```python
from build123d import *

# Parameters (mm, degrees)
BOSS_EXTRUDE1_DEPTH      = 4
BOSS_EXTRUDE1_DEPTH_BACK = 4
SKETCH3_W                = 89.310018428
SKETCH3_H                = 59.716622104
BOSS_EXTRUDE2_DEPTH      = 4
CUT_EXTRUDE1_REACH       = 112.584
SKETCH4_R                = 2.25
SKETCH5_W                = 83.9215243
SKETCH5_H                = 34.4
BOSS_EXTRUDE3_DEPTH      = 4
SKETCH6_R                = 2.25
CUT_EXTRUDE2_DEPTH       = 4
FILLET1_R                = 5
SKETCH7_R                = 2.1
CUT_EXTRUDE3_DEPTH       = 109.665502377


with BuildPart() as part:
    # Sketch2 → Boss-Extrude1 (new, two sides: drawn at the far end of the back side and taken through both)
    with BuildSketch(Plane(origin=(0, 0, 0), x_dir=(1, 0, 0), z_dir=(0, 1, 0)).offset(-BOSS_EXTRUDE1_DEPTH_BACK)):
        with BuildLine():
            Line((1.154700538, 0), (85.076224838, 0))
            ThreePointArc((85.076224838, 0), (82.329376533, -33.6502282), (67.376468713, -63.920569811))
            Line((67.376468713, -63.920569811), (-9.968276059, -19.265560597))
            Line((-9.968276059, -19.265560597), (1.154700538, 0))
        make_face()
    extrude(amount=BOSS_EXTRUDE1_DEPTH + BOSS_EXTRUDE1_DEPTH_BACK)

    # Sketch3 → Boss-Extrude2 (add)
    with BuildSketch(Plane(origin=(-10.834301462, 0, 18.765560597), x_dir=(0.8660254037844386, 0, 0.5000000000000001), z_dir=(-0.5000000000000001, 0, 0.8660254037844386))):
        with Locations((45.655009214, 0)):
            Rectangle(SKETCH3_W, SKETCH3_H)
    extrude(amount=-BOSS_EXTRUDE2_DEPTH)

    # Sketch4 → Cut-Extrude1 (cut, up to next)
    with BuildSketch(Plane(origin=(-10.834301462, 0, 18.765560597), x_dir=(0.8660254037844386, 0, 0.5000000000000001), z_dir=(-0.5000000000000001, 0, 0.8660254037844386)), mode=Mode.PRIVATE) as cut_extrude1_sk1:
        with Locations((66, 21.858311052)):
            Circle(SKETCH4_R)
    cut_extrude1_tool1 = extrude(cut_extrude1_sk1.sketch, amount=-CUT_EXTRUDE1_REACH, mode=Mode.PRIVATE) & part.part
    # Sketch4 → Cut-Extrude1 (cut, up to next)
    with BuildSketch(Plane(origin=(-10.834301462, 0, 18.765560597), x_dir=(0.8660254037844386, 0, 0.5000000000000001), z_dir=(-0.5000000000000001, 0, 0.8660254037844386)), mode=Mode.PRIVATE) as cut_extrude1_sk2:
        with Locations((66, -21.858311052)):
            Circle(SKETCH4_R)
    cut_extrude1_tool2 = extrude(cut_extrude1_sk2.sketch, amount=-CUT_EXTRUDE1_REACH, mode=Mode.PRIVATE) & part.part
    # Sketch4 → Cut-Extrude1 (cut, up to next)
    with BuildSketch(Plane(origin=(-10.834301462, 0, 18.765560597), x_dir=(0.8660254037844386, 0, 0.5000000000000001), z_dir=(-0.5000000000000001, 0, 0.8660254037844386)), mode=Mode.PRIVATE) as cut_extrude1_sk3:
        with Locations((18.5, 21.858311052)):
            Circle(SKETCH4_R)
    cut_extrude1_tool3 = extrude(cut_extrude1_sk3.sketch, amount=-CUT_EXTRUDE1_REACH, mode=Mode.PRIVATE) & part.part
    # Sketch4 → Cut-Extrude1 (cut, up to next)
    with BuildSketch(Plane(origin=(-10.834301462, 0, 18.765560597), x_dir=(0.8660254037844386, 0, 0.5000000000000001), z_dir=(-0.5000000000000001, 0, 0.8660254037844386)), mode=Mode.PRIVATE) as cut_extrude1_sk4:
        with Locations((18.5, -21.858311052)):
            Circle(SKETCH4_R)
    cut_extrude1_tool4 = extrude(cut_extrude1_sk4.sketch, amount=-CUT_EXTRUDE1_REACH, mode=Mode.PRIVATE) & part.part
    add(cut_extrude1_tool1.solids().sort_by_distance((46.323375, 21.858311, 51.765561))[0], mode=Mode.SUBTRACT)
    add(cut_extrude1_tool2.solids().sort_by_distance((46.323375, -21.858311, 51.765561))[0], mode=Mode.SUBTRACT)
    add(cut_extrude1_tool3.solids().sort_by_distance((5.187169, 21.858311, 28.015561))[0], mode=Mode.SUBTRACT)
    add(cut_extrude1_tool4.solids().sort_by_distance((5.187169, -21.858311, 28.015561))[0], mode=Mode.SUBTRACT)

    # Sketch5 → Boss-Extrude3 (add)
    with BuildSketch(Plane(origin=(0, 0, 0), x_dir=(-1, 0, 0), z_dir=(0, 0, -1))):
        with Locations((-43.115462688, 0)):
            Rectangle(SKETCH5_W, SKETCH5_H)
    extrude(amount=-BOSS_EXTRUDE3_DEPTH)

    # Sketch6 → Cut-Extrude2 (cut)
    with BuildSketch(Plane(origin=(0, 0, 0), x_dir=(-1, 0, 0), z_dir=(0, 0, -1))):
        with Locations((-71.25, -9.2)):
            Circle(SKETCH6_R)
        with Locations((-71.25, 9.2)):
            Circle(SKETCH6_R)
        with Locations((-42.75, 9.2)):
            Circle(SKETCH6_R)
        with Locations((-42.75, -9.2)):
            Circle(SKETCH6_R)
    extrude(amount=-CUT_EXTRUDE2_DEPTH, mode=Mode.SUBTRACT)

    # Fillet1
    fillet1_edges = [part.edges().sort_by_distance(p)[0] for p in [
        (30.704096327, 4, 38.128963589),
        (30.704096327, -4, 38.128963589),
    ]]
    fillet(fillet1_edges, radius=FILLET1_R)

    # Sketch7 → Cut-Extrude3 (cut, through all)
    with BuildSketch(Plane.XY.offset(4)):
        with Locations(Location((42.75, 9.2, 0), (0, 0, 180))):
            Circle(SKETCH7_R)
        with Locations((71.25, 9.2)):
            Circle(SKETCH7_R)
    cut_extrude3 = extrude(amount=CUT_EXTRUDE3_DEPTH, mode=Mode.SUBTRACT)

    # Mirror1: Cut-Extrude3 across plane
    add(cut_extrude3.mirror(Plane.ZX), mode=Mode.SUBTRACT)


solid = part.part
```
Read the model definition and answer for the solid it produces. Units are mm, in the model's axes. A direction names the side the tool comes from. Coordinates: 2 decimals unless noted, no trailing zeros. Loops run counter-clockwise (first coordinate to the right, second up) from the corner with the lowest first, then second, coordinate; pieces in that order, holes last.
(1) Consider line 1 along Y through (x, z) = (71.25, 2.35); line 2 along Y through (x, z) = (42.75, 48.25); line 3 along X through (y, z) = (-9, 2). Determine where each line is inside the solid, lowest interval first.
Solution:
line 1: y = -17.2 to -11.45, -6.95 to 6.95, 11.45 to 17.2
line 2: y = -29.86 to -11.3, -7.1 to 7.1, 11.3 to 29.86
line 3: x = 1.15 to 40.51, 44.99 to 69.01, 73.49 to 85.08
(2) The part is cut by section A-A (y = 12.5). Determine the outline of the cut face in (x, z), and give its area (3 significant figures).
Solution:
outline: (-9.97, 19.27) - (-7.97, 15.8) - (69.38, 60.46) - (67.38, 63.92) - close; (1.15, 0) - (85.08, 0) - (85.08, 4) - (1.15, 4) - close
area: 693 mm2
(3) The part is cut by section C-C (z = 7). Determine the outline of the cut face in (x, y).
Solution:
outline: (-2.89, -4) - (85.55, -4) - (85.55, 4) - (-2.89, 4) - close
(4) The part is cut by section D-D (x = 42.75). Count the separate pieces of the cut face and the enclosed holes in it, and give its area (3 significant figures).
Solution:
separate pieces: 5
enclosed holes: 0
area: 679 mm2
(5) Flat-ended cylindrical pins translate along their axes: pin 1 Ø4 at (x, y) = (71.25, -9.2) entering from +Z; pin 2 Ø10 at (y, z) = (-18, 54) entering from +X; pin 3 Ø4 at (y, z) = (-8, 16.5) entering from +X; pin 4 Ø3 at (y, z) = (11, 2.5) entering from +X. Find the tip coordinate at first contact, or state that the pin passes through.
Solution:
pin 1: passes through
pin 2: stops at x = 66.85
pin 3: stops at x = -2.91
pin 4: stops at x = 85.08
(6) The part is cut by section B-B (x = 78). Determine the outline of the cut face in (y, z), and give its area (3 significant figures).
Solution:
outline: (-17.2, 0) - (17.2, 0) - (17.2, 4) - (4, 4) - (4, 45.81) - (-4, 45.81) - (-4, 4) - (-17.2, 4) - close
area: 472 mm2
(7) The mould has two halves that part along Z. Classify faces 6 (the face through (44, 0, 0)), 7 (the face through (30.914, -5.426, 36.514)), 8 (the face through (51, -4, 24)), 9 (the face through (68.6, 16.7, 61.8)): released by +Z, released by -Z, zero draft, split by the parting line, or undercut.
Solution:
face 6: released by -Z
face 7: undercut
face 8: undercut
face 9: released by +Z
(8) A tool of negligible diameter and unlimited length cuts with its end or side. For faces 1 (the face through (85.076, -11, 2)), 2 (the face through (69.17, -10.06, 1.97)), 3 (the face through (44, -12, 4)), 4 (the face through (85.076, 11, 2)), 5 (the face through (44, -17.2, 2)), from which of +Z, -Z, +X, -X, +Y, -Y can it reach the whole face along a straight path? Write none if from no direction.
Solution:
face 1: +Z, -Z, +X, -Y
face 2: -Z
face 3: +X, -X, -Y
face 4: +Z, -Z, +X, +Y
face 5: -Z, +X, -X, -Y
